```python
from build123d import *

# Parameters (mm, degrees)
Y_KSEKLIK_EKSTR_ZYON1_DEPTH = 100


with BuildPart() as part:
    # Çizim1 → Yükseklik-Ekstrüzyon1 (new body)
    with BuildSketch(Plane.XY.offset(100)):
        with BuildLine():
            Line((5, -21), (6, -21))
            Line((6, -21), (6, -22.5))
            Line((6, -22.5), (19.5, -22.5))
            ThreePointArc((19.5, -22.5), (21.621320344, -21.621320344), (22.5, -19.5))
            Line((22.5, -19.5), (22.5, -6))
            Line((22.5, -6), (21, -6))
            Line((21, -6), (21, -5))
            Line((21, -5), (16.499999999, -5))
            Line((16.499999999, -5), (16.499999999, -10.000000002))
            Line((16.499999999, -10.000000002), (11.979898986, -10.000000002))
            Line((11.979898986, -10.000000002), (7.27644295, -5.296543966))
            ThreePointArc((7.27644295, -5.296543966), (8.999999998, -2e-09), (7.27644295, 5.296543963))
            Line((7.27644295, 5.296543963), (11.979898987, 10))
            Line((11.979898987, 10), (16.499999999, 10))
            Line((16.499999999, 10), (16.499999999, 5))
            Line((16.499999999, 5), (21, 5))
            Line((21, 5), (21, 6))
            Line((21, 6), (22.5, 6))
            Line((22.5, 6), (22.5, 19.5))
            ThreePointArc((22.5, 19.5), (21.621320344, 21.621320344), (19.5, 22.5))
            Line((19.5, 22.5), (6, 22.5))
            Line((6, 22.5), (6, 21))
            Line((6, 21), (5, 21))
            Line((5, 21), (5, 16.499999998))
            Line((5, 16.499999998), (10, 16.499999998))
            Line((10, 16.499999998), (10, 11.979898987))
            Line((10, 11.979898987), (5.296543963, 7.27644295))
            ThreePointArc((5.296543963, 7.27644295), (-2e-09, 8.999999998), (-5.296543966, 7.27644295))
            Line((-5.296543966, 7.27644295), (-10.000000001, 11.979898985))
            Line((-10.000000001, 11.979898985), (-10.000000001, 16.499999998))
            Line((-10.000000001, 16.499999998), (-5, 16.499999998))
            Line((-5, 16.499999998), (-5, 21))
            Line((-5, 21), (-6, 21))
            Line((-6, 21), (-6, 22.5))
            Line((-6, 22.5), (-19.5, 22.5))
            ThreePointArc((-19.5, 22.5), (-21.621320344, 21.621320344), (-22.5, 19.5))
            Line((-22.5, 19.5), (-22.5, 6))
            Line((-22.5, 6), (-21, 6))
            Line((-21, 6), (-21, 5))
            Line((-21, 5), (-16.500000001, 5))
            Line((-16.500000001, 5), (-16.500000001, 10))
            Line((-16.500000001, 10), (-11.979898987, 10))
            Line((-11.979898987, 10), (-7.276442952, 5.296543965))
            ThreePointArc((-7.276442952, 5.296543965), (-9.000000001, -1e-09), (-7.276442953, -5.296543966))
            Line((-7.276442953, -5.296543966), (-11.979898988, -10.000000002))
            Line((-11.979898988, -10.000000002), (-16.500000001, -10.000000002))
            Line((-16.500000001, -10.000000002), (-16.500000001, -5))
            Line((-16.500000001, -5), (-21, -5))
            Line((-21, -5), (-21, -6))
            Line((-21, -6), (-22.5, -6))
            Line((-22.5, -6), (-22.5, -19.5))
            ThreePointArc((-22.5, -19.5), (-21.621320344, -21.621320344), (-19.5, -22.5))
            Line((-19.5, -22.5), (-6, -22.5))
            Line((-6, -22.5), (-6, -21))
            Line((-6, -21), (-5, -21))
            Line((-5, -21), (-5, -16.500000002))
            Line((-5, -16.500000002), (-10.000000001, -16.500000002))
            Line((-10.000000001, -16.500000002), (-10.000000001, -11.979898989))
            Line((-10.000000001, -11.979898989), (-5.296543966, -7.276442954))
            ThreePointArc((-5.296543966, -7.276442954), (0, -9.000000002), (5.296543965, -7.276442952))
            Line((5.296543965, -7.276442952), (10, -11.979898987))
            Line((10, -11.979898987), (10, -16.500000002))
            Line((10, -16.500000002), (5, -16.500000002))
            Line((5, -16.500000002), (5, -21))
        make_face()
        Polygon((-11.98, 18.500101013), (-11.98, 11.98), (-18.500101013, 11.98), (-18.500101013, 7.000101013), (-20.500101013, 7.000101013), (-20.500101013, 20.500101013), (-7.000101013, 20.500101013), (-7.000101013, 18.500101013), align=None, mode=Mode.SUBTRACT)
        Polygon((-18.500101013, -11.98), (-11.98, -11.98), (-11.98, -18.500101013), (-7.000101013, -18.500101013), (-7.000101013, -20.500101013), (-20.500101013, -20.500101013), (-20.500101013, -7.000101013), (-18.500101013, -7.000101013), align=None, mode=Mode.SUBTRACT)
        Polygon((11.98, -18.500101013), (11.98, -11.98), (18.500101013, -11.98), (18.500101013, -7.000101013), (20.500101013, -7.000101013), (20.500101013, -20.500101013), (7.000101013, -20.500101013), (7.000101013, -18.500101013), align=None, mode=Mode.SUBTRACT)
        Polygon((18.500101013, 11.98), (11.98, 11.98), (11.98, 18.500101013), (7.000101013, 18.500101013), (7.000101013, 20.500101013), (20.500101013, 20.500101013), (20.500101013, 7.000101013), (18.500101013, 7.000101013), align=None, mode=Mode.SUBTRACT)
        with BuildLine():
            Line((-6.52021344, -4.635387443), (-4.075133401, -2.897117152))
            ThreePointArc((-4.075133401, -2.897117152), (-4.635428757, -1.874246585), (-4.943520618, -0.749402378))
            Line((-4.943520618, -0.749402378), (-5.932224741, -0.899282854))
            ThreePointArc((-5.932224741, -0.899282854), (-6.000000002, -2e-09), (-5.932224741, 0.89928285))
            Line((-5.932224741, 0.89928285), (-4.943520618, 0.749402375))
            ThreePointArc((-4.943520618, 0.749402375), (-4.635428757, 1.874246582), (-4.0751334, 2.89711715))
            Line((-4.0751334, 2.89711715), (-6.520213439, 4.635387441))
            ThreePointArc((-6.520213439, 4.635387441), (-5.65685425, 5.656854249), (-4.635387441, 6.520213437))
            Line((-4.635387441, 6.520213437), (-2.897117152, 4.075133398))
            ThreePointArc((-2.897117152, 4.075133398), (-1.874246584, 4.635428754), (-0.749402378, 4.943520614))
            Line((-0.749402378, 4.943520614), (-0.899282853, 5.932224737))
            ThreePointArc((-0.899282853, 5.932224737), (-5e-09, 5.999999998), (0.899282844, 5.932224738))
            Line((0.899282844, 5.932224738), (0.74940237, 4.943520615))
            ThreePointArc((0.74940237, 4.943520615), (1.874246579, 4.635428755), (2.897117149, 4.075133397))
            Line((2.897117149, 4.075133397), (4.635387439, 6.520213436))
            ThreePointArc((4.635387439, 6.520213436), (5.656854248, 5.656854248), (6.520213436, 4.635387439))
            Line((6.520213436, 4.635387439), (4.075133397, 2.897117149))
            ThreePointArc((4.075133397, 2.897117149), (4.635428754, 1.874246581), (4.943520614, 0.749402374))
            Line((4.943520614, 0.749402374), (5.932224737, 0.89928285))
            ThreePointArc((5.932224737, 0.89928285), (5.999999998, -2e-09), (5.932224737, -0.899282854))
            Line((5.932224737, -0.899282854), (4.943520614, -0.749402379))
            ThreePointArc((4.943520614, -0.749402379), (4.635428753, -1.874246586), (4.075133396, -2.897117154))
            Line((4.075133396, -2.897117154), (6.520213435, -4.635387445))
            ThreePointArc((6.520213435, -4.635387445), (5.656854247, -5.656854253), (4.635387438, -6.520213441))
            Line((4.635387438, -6.520213441), (2.897117148, -4.075133401))
            ThreePointArc((2.897117148, -4.075133401), (1.874246581, -4.635428758), (0.749402374, -4.943520618))
            Line((0.749402374, -4.943520618), (0.899282849, -5.932224741))
            ThreePointArc((0.899282849, -5.932224741), (1e-09, -6.000000002), (-0.899282847, -5.932224742))
            Line((-0.899282847, -5.932224742), (-0.749402373, -4.943520619))
            ThreePointArc((-0.749402373, -4.943520619), (-1.874246583, -4.635428758), (-2.897117153, -4.075133401))
            Line((-2.897117153, -4.075133401), (-4.635387443, -6.52021344))
            ThreePointArc((-4.635387443, -6.52021344), (-5.656854252, -5.656854251), (-6.52021344, -4.635387443))
        make_face(mode=Mode.SUBTRACT)
    extrude(amount=-Y_KSEKLIK_EKSTR_ZYON1_DEPTH)


solid = part.part
```
The listing builds one solid part. Answer for the finished solid, in the listing's coordinates (mm). A direction names the side the tool comes from. Give positions to 0.01 mm unless a question says otherwise; leave off trailing zeros. Order: outer loops, then holes, each group sorted by start corner. A loop starts at its lowest first (then second) coordinate and runs counter-clockwise, first axis right, second up. Notation, with made-up numbers: (30, 16.5) -> (88, 16.5) arc R19 cw to (88, 48.5) -> close; hole circle Ø9 at (56, -4). An arc over 180 degrees is marked (long way). Answer as a JSON object with one key per item and string values. Group by question number.
Item 1: The part is cut by section A-A on x = -15.5. Write down the section's boundary in (y, z).
Item 2: Determine the mould class of faces 4 (the flat face through (16.5, -7, 51)), 5 (the flat face through (7, 19, 51)) for opening direction X: pulls with the +X half, pulls with the -X half, needs draft (parallel to the pull), parting line crosses it, or undercut.
Item 3: The part is cut by section B-B on z = 42.5. Give the number of separate pieces and of enclosed holes in the cut face, and give its area (3 significant figures).
Item 4: A flat-ended cylindrical pin translates along its axis: pin 1 (1.6 mm diameter, centred on y = 21.5, z = 47, fed in from -X). Find the tip coordinate at first contact, or state that the pin passes through.
Item 5: A tool of negligible diameter and unlimited length cuts with its end or side. For faces 1 (the flat face through (5, -19, 51)), 2 (the flat face through (5, 19, 51)), 3 (the cylindrical face through (5.644, 5.67, 50.7)), from which of +Z, -Z, +X, -X, +Y, -Y can it reach the whole face along a straight path? Write none if from no direction.
Item 6: Consider L1, parallel to X at y = 18, z = 87.5; L2, parallel to X at y = 14, z = 42. Determine where each line is inside the solid, lowest interval first. Write a range as from..to.
Result set:
{
 "1": {"outline": "(-22.5, 0) -> (-20.5, 0) -> (-20.5, 100) -> (-22.5, 100) -> close; (-11.98, 0) -> (-10, 0) -> (-10, 100) -> (-11.98, 100) -> close; (10, 0) -> (11.98, 0) -> (11.98, 100) -> (10, 100) -> close; (20.5, 0) -> (22.5, 0) -> (22.5, 100) -> (20.5, 100) -> close"},
 "2": {"face 4": "undercut", "face 5": "undercut"},
 "3": {"separate pieces": "1", "enclosed holes": "5", "area": "684 mm²"},
 "4": {"pin 1": "x = -22.25"},
 "5": {"face 1": "+Z, -Z, -Y", "face 2": "+Z, -Z, +Y", "face 3": "+Z, -Z"},
 "6": {"L1": "-22.5..-20.5, -11.98..-5, 5..11.98, 20.5..22.5", "L2": "-22.5..-20.5, -11.98..-10, 10..11.98, 20.5..22.5"}
}
